Verification items for the finished model (mm, model axes). Give positions to 0.01 mm unless a question says otherwise; leave off trailing zeros. Loops run counter-clockwise (first coordinate to the right, second up) from the corner with the lowest first, then second, coordinate; pieces in that order, holes last. Notation, with made-up numbers: M 25,-3 L 38,-3 A18 cw 38,26 Z; hole C 23,-21.5 d5. An arc over 180 degrees is marked long. Use CSV: the item, a comma, the result in double quotes.
from build123d import *

# Parameters (mm, degrees)
SKETCH1_W                = 20
SKETCH1_H                = 40
BOSS_EXTRUDE1_DEPTH      = 1.3
M3_CLEARANCE_HOLE1_D     = 3.4
M3_CLEARANCE_HOLE1_DEPTH = 1.3
FILLET1_R                = 2.5


with BuildPart() as part:
    # Sketch1 → Boss-Extrude1 (new body)
    with BuildSketch(Plane(origin=(0, 0, 0), x_dir=(1, 0, 0), z_dir=(0, 1, 0))):
        with Locations((10, -20)):
            Rectangle(SKETCH1_W, SKETCH1_H)
    extrude(amount=BOSS_EXTRUDE1_DEPTH)

    # M3 Clearance Hole1
    with Locations(Plane(origin=(0, 1.3, 0), x_dir=(1, 0, 0), z_dir=(0, 1, 0))):
        with Locations((10, -5.5)):
            Hole(M3_CLEARANCE_HOLE1_D / 2, depth=M3_CLEARANCE_HOLE1_DEPTH)

    # Fillet1
    fillet1_edges = [part.edges().sort_by_distance(p)[0] for p in [
        (0, 0.65, 0),
        (20, 0.65, 0),
        (20, 0.65, 40),
        (0, 0.65, 40),
    ]]
    fillet(fillet1_edges, radius=FILLET1_R)


solid = part.part
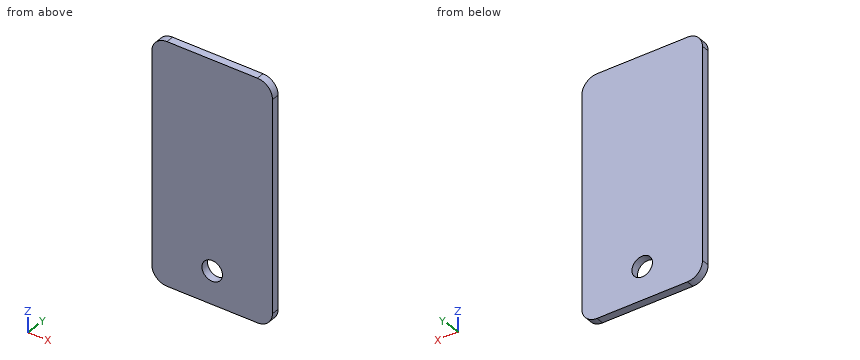
(1) Scan lines: L1, parallel to X at y = 0.8, z = 5.5; L2, parallel to Z at x = 10, y = 1; L3, parallel to Z at x = 10.5, y = 0.35. Record each from-to range of solid material in increasing order. Write a range as from..to.
Calculated:
L1,"x = 0..8.3, 11.7..20"
L2,"z = 0..3.8, 7.2..40"
L3,"z = 0..3.88, 7.12..40"
(2) Section check B-B on x = 10. Record the cut outline in (y, z), plus the area to 3 significant figures.
Calculated:
outline,"M 0,0 L 1.3,0 L 1.3,3.8 L 0,3.8 Z; M 0,7.2 L 1.3,7.2 L 1.3,40 L 0,40 Z"
area,"47.6 mm²"
(3) Section check A-A on y = 0.35. Record the cut outline in (x, z).
Calculated:
outline,"M 0,2.5 A2.5 ccw 2.5,0 L 17.5,0 A2.5 ccw 20,2.5 L 20,37.5 A2.5 ccw 17.5,40 L 2.5,40 A2.5 ccw 0,37.5 Z; hole C 10,5.5 d3.4"
(4) Section check C-C on z = 5.5. Record the cut outline in (x, y), plus the area to 3 significant figures.
Calculated:
outline,"M 0,0 L 8.3,0 L 8.3,1.3 L 0,1.3 Z; M 11.7,0 L 20,0 L 20,1.3 L 11.7,1.3 Z"
area,"21.6 mm²"
